from build123d import *

# Parameters (mm, degrees)
BOSS_EXTRUDE1_DEPTH = 10
CUT_EXTRUDE3_REACH  = 13.51
SKETCH2_R           = 2


with BuildPart() as part:
    # Sketch1 → Boss-Extrude1 (new body)
    with BuildSketch(Plane.XY):
        with BuildLine():
            Line((8.4952987, 0.5), (18.5, 0.5))
            Line((18.5, 0.5), (18.5, 3.500157096))
            Line((18.5, 3.500157096), (10.964898554, 3.500157096))
            ThreePointArc((10.964898554, 3.500157096), (0, 11.51), (-10.964898554, 3.500157096))
            Line((-10.964898554, 3.500157096), (-18.5, 3.500157096))
            Line((-18.5, 3.500157096), (-18.5, 0.5))
            Line((-18.5, 0.5), (-8.4952987, 0.5))
            ThreePointArc((-8.4952987, 0.5), (0, 8.51), (8.4952987, 0.5))
        make_face()
    extrude(amount=BOSS_EXTRUDE1_DEPTH)

    # Sketch2 → Cut-Extrude3 (cut, up to next)
    with BuildSketch(Plane(origin=(0, 0, 0), x_dir=(1, 0, 0), z_dir=(0, 1, 0)), mode=Mode.PRIVATE) as cut_extrude3_sk1:
        with Locations((-14.732448989, -5)):
            Circle(SKETCH2_R)
    cut_extrude3_tool1 = extrude(cut_extrude3_sk1.sketch, amount=CUT_EXTRUDE3_REACH, mode=Mode.PRIVATE) & part.part
    add(cut_extrude3_tool1.solids().sort_by_distance((-14.732449, 0, 5))[0], mode=Mode.SUBTRACT)
    # Sketch2 → Cut-Extrude3 (cut, up to next)
    with BuildSketch(Plane(origin=(0, 0, 0), x_dir=(1, 0, 0), z_dir=(0, 1, 0)), mode=Mode.PRIVATE) as cut_extrude3_sk2:
        with Locations((14.732448989, -5)):
            Circle(SKETCH2_R)
    cut_extrude3_tool2 = extrude(cut_extrude3_sk2.sketch, amount=CUT_EXTRUDE3_REACH, mode=Mode.PRIVATE) & part.part
    add(cut_extrude3_tool2.solids().sort_by_distance((14.732449, 0, 5))[0], mode=Mode.SUBTRACT)


solid = part.part
For this review, take the finished solid that the model builds, in its own axes (mm). A direction names the side the tool comes from. Round coordinates to 2 decimals unless told otherwise and drop trailing zeros. Order: outer loops, then holes, each group sorted by start corner. A loop starts at its lowest first (then second) coordinate and runs counter-clockwise, first axis right, second up. Notation, with made-up numbers: M 48.25,84.5 L 71.25,84.5 A29 cw 71.25,109.5 Z; hole C -27.75,42 d8. An arc over 180 degrees is marked long. Use a Markdown table: item, result. Add a question column.
Item 1: Tool access review of faces 1 (the flat face through (-14.7, 3.5, 2.7)), 2 (the flat face through (18.5, 2, 5)): name each direction out of +Z, -Z, +X, -X, +Y, -Y from which nothing blocks a thin tool from reaching the whole face with its end or side.
Item 2: Add section C-C, the plane y = 1.75. Give the boundary of the cut face in (x, z), then the cut area to 3 significant figures.
Item 3: Insertion check: pin 1 (6 mm diameter, centred on x = -16.5, z = 3, fed in from +Y); pin 2 (6 mm diameter, centred on x = 1, y = 2.5, fed in from -Z); pin 3 (1.5 mm diameter, centred on y = 8.5, z = 7, fed in from -X); pin 4 (1.5 mm diameter, centred on x = 9, z = 8, fed in from +Y). Each pin has a flat end and moves straight along its axis. Give the tip position at first contact, or say it passes through.
Item 4: Add section B-B, the plane y = 7.5. Give the boundary of the cut face in (x, z), then the cut area to 3 significant figures.
Item 5: Mouldability with a two-part tool opening along X and no side actions: class faces 3 (the cylindrical face through (0.2, 11.51, 4.93)), 4 (the flat face through (14.8, 3.5, 2.7)), 5 (the cylindrical face through (16.58, 1.98, 5.77)) as released by +X, released by -X, zero draft, split by the parting line, or undercut.
Item 6: To check wall thickness, follow line 1 along X through (y, z) = (1.75, 6.25); line 2 along Y through (x, z) = (15.5, 7.75); line 3 along X through (y, z) = (7.25, 4.75). State the ranges of each line that lie inside material, in increasing order.
Item 7: Add section D-D, the plane x = 0. Give the boundary of the cut face in (y, z), then the cut area to 3 significant figures.
Geometry results:
| question | item | result |
|---|---|---|
| 1 | face 1 | +Z, -Z, -X, +Y |
| 1 | face 2 | +Z, -Z, +X, +Y, -Y |
| 2 | outline | M -18.5,0 L -8.33,0 L -8.33,10 L -18.5,10 Z; M 8.33,0 L 18.5,0 L 18.5,10 L 8.33,10 Z; hole C -14.73,5 d4; hole C 14.73,5 d4 |
| 2 | area | 178 mm² |
| 3 | pin 1 | stops at y = 3.5 |
| 3 | pin 2 | passes through |
| 3 | pin 3 | stops at x = -8.51 |
| 3 | pin 4 | stops at y = 8.03 |
| 4 | outline | M -8.73,0 L -4.02,0 L -4.02,10 L -8.73,10 Z; M 4.02,0 L 8.73,0 L 8.73,10 L 4.02,10 Z |
| 4 | area | 94.2 mm² |
| 5 | face 3 | split by the parting line |
| 5 | face 4 | zero draft |
| 5 | face 5 | undercut |
| 6 | line 1 | x = -18.5 to -16.29, -13.17 to -8.33, 8.33 to 13.17, 16.29 to 18.5 |
| 6 | line 2 | y = 0.5 to 3.5 |
| 6 | line 3 | x = -8.94 to -4.46, 4.46 to 8.94 |
| 7 | outline | M 8.51,0 L 11.51,0 L 11.51,10 L 8.51,10 Z |
| 7 | area | 30.0 mm² |
